Can you work these out from the model? Positions are in its coordinate system, mm. Face numbers are marked on the shaded views. A direction names the side the tool comes from. Round coordinates to 2 decimals unless told otherwise and drop trailing zeros. Order: outer loops, then holes, each group sorted by start corner. A loop starts at its lowest first (then second) coordinate and runs counter-clockwise, first axis right, second up.
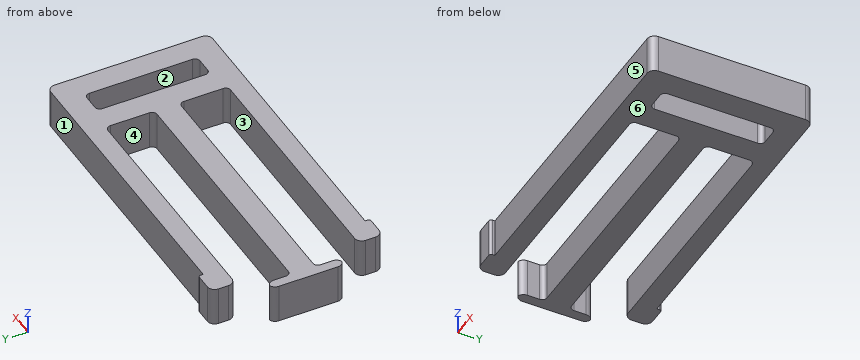
from build123d import *

# Parameters (mm, degrees)
SKETCH1_W           = 23
SKETCH1_H           = 5
BOSS_EXTRUDE2_DEPTH = 8
FILLET1_R           = 1
FILLET2_R           = 0.5
FILLET3_R           = 1.5


with BuildPart() as part:
    # Sketch1 → Boss-Extrude2 (new body)
    with BuildSketch(Plane(origin=(0, 0, 0), x_dir=(0, 1, 0), z_dir=(0, 0, 1))):
        Polygon((0, 0), (-33, 0), (-33, 60.6), (-34, 60.6), (-34, 65.6), (-29, 65.6), (-29, 15), (-19, 15), (-19, 68), (-24, 68), (-24, 70), (-9, 70), (-9, 68), (-14, 68), (-14, 15), (-4, 15), (-4, 65.6), (1, 65.6), (1, 60.6), (0, 60.6), align=None)
        with Locations((-16.5, 7.5)):
            Rectangle(SKETCH1_W, SKETCH1_H, mode=Mode.SUBTRACT)
    extrude(amount=BOSS_EXTRUDE2_DEPTH)

    # Fillet1
    fillet1_edges = [part.edges().sort_by_distance(p)[0] for p in [
        (-15, -29, 4),
        (-15, -19, 4),
        (-68, -19, 4),
        (-68, -14, 4),
        (-15, -14, 4),
        (-15, -4, 4),
        (-10, -5, 4),
        (-10, -28, 4),
        (-5, -28, 4),
        (-5, -5, 4),
    ]]
    fillet(fillet1_edges, radius=FILLET1_R)

    # Fillet2
    fillet2_edges = [part.edges().sort_by_distance(p)[0] for p in [
        (-60.6, -34, 4),
        (-60.6, 1, 4),
    ]]
    fillet(fillet2_edges, radius=FILLET2_R)

    # Fillet3
    # the kernel refuses this fillet: 1.5 mm, written as the material it takes off along each edge
    with BuildSketch(Plane(origin=(-70, -24, -3.75), x_dir=(1, 0, 0), z_dir=(0, 0, 1)), Plane(origin=(-70, -9, -3.75), x_dir=(0, -1, 0), z_dir=(0, 0, 1)), Plane(origin=(-68, -9, -3.75), x_dir=(-1, 0, 0), z_dir=(0, 0, 1)), Plane(origin=(-68, -24, -3.75), x_dir=(0, 1, 0), z_dir=(0, 0, 1)), Plane(origin=(-65.6, -29, -3.75), x_dir=(0, -1, 0), z_dir=(0, 0, 1)), Plane(origin=(-65.6, -34, -3.75), x_dir=(1, 0, 0), z_dir=(0, 0, 1))) as fillet3_piece_1:
        with BuildLine():
            CenterArc((FILLET3_R, FILLET3_R), FILLET3_R, 180, 90)
            Line((0, FILLET3_R), (0, 0))
            Line((0, 0), (FILLET3_R, 0))
        make_face()
    extrude(amount=15.5, mode=Mode.SUBTRACT)
    with BuildSketch(Plane(origin=(0, -33, -3.75), x_dir=(-1, 0, 0), z_dir=(0, 0, 1)), Plane(origin=(0, 0, -3.75), x_dir=(0, -1, 0), z_dir=(0, 0, 1)), Plane(origin=(-65.6, 1, -3.75), x_dir=(1, 0, 0), z_dir=(0, 0, 1)), Plane(origin=(-65.6, -4, -3.75), x_dir=(0, 1, 0), z_dir=(0, 0, 1))) as fillet3_piece_2:
        with BuildLine():
            CenterArc((FILLET3_R, -FILLET3_R), FILLET3_R, 90, 90)
            Line((0, -FILLET3_R), (0, 0))
            Line((0, 0), (FILLET3_R, 0))
        make_face()
    extrude(amount=15.5, mode=Mode.SUBTRACT)


solid = part.part
(1) If we mould it in two halves opening along Y, with no side actions, what happens to the marked faces 4, 5 and 6? For each: pulls with the +Y half, pulls with the -Y half, needs draft (parallel to the pull), parting line crosses it, or undercut.
(2) I'm going to push flat-ended pins straight in: pin 1 Ø1.5 at (x, z) = (-15, 7) entering from -Y; pin 2 Ø1 at (y, z) = (-32, 3.5) entering from -X; pin 3 Ø3 at (x, y) = (-15, -5) entering from -Z; pin 4 Ø2.5 at (x, z) = (-43, 3) entering from +Y. Where does each tip first touch, or does it pass through?
(3) I want a section at B-B, the plane y = -25.5. List the corners of the cut face in (x, z) for me, plus the area to 3 significant figures.
(4) On a 3-axis mill with a long thin cutter (end or side, diameter ignored), from which of +Z, -Z, +X, -X, +Y, -Y can I reach the whole of each face in a straight line? I mean the marked faces 1, 2 and 3. Say none if no direction works.
(5) Please list where these lines run through material, in increasing order: probe 1 along Y at (x, z) = (-25.5, 5.5); probe 2 along X at (y, z) = (-12.5, 7.5); probe 3 along Y at (x, z) = (-61, 0.5).
(6) I want a section at A-A, the plane y = -21. List the corners of the cut face in (x, z) for me.
(7) I want a section at C-C, the plane x = -41. List the corners of the cut face in (y, z) for me.
Ans:
1. face 4: undercut
1. face 5: pulls with the -Y half
1. face 6: needs draft
2. pin 1: stops at y = -33
2. pin 2: stops at x = -65.6
2. pin 3: stops at z = 0
2. pin 4: stops at y = 0
3. outline: (-15, 0) - (-10, 0) - (-10, 8) - (-15, 8) - close; (-5, 0) - (0, 0) - (0, 8) - (-5, 8) - close
3. area: 80.0 mm2
4. face 1: +Z, -Z, +X, +Y
4. face 2: +Z, -Z
4. face 3: +Z, -Z, -X
5. probe 1: y = -33 to -29, -19 to -14, -4 to 0
5. probe 2: x = -70 to -68, -15 to -10, -5 to 0
5. probe 3: y = -33.99 to -29, -19 to -14, -4 to 0.99
6. outline: (-70, 0) - (-68, 0) - (-68, 8) - (-70, 8) - close; (-15, 0) - (-10, 0) - (-10, 8) - (-15, 8) - close; (-5, 0) - (0, 0) - (0, 8) - (-5, 8) - close
7. outline: (-33, 0) - (-29, 0) - (-29, 8) - (-33, 8) - close; (-19, 0) - (-14, 0) - (-14, 8) - (-19, 8) - close; (-4, 0) - (0, 0) - (0, 8) - (-4, 8) - close
